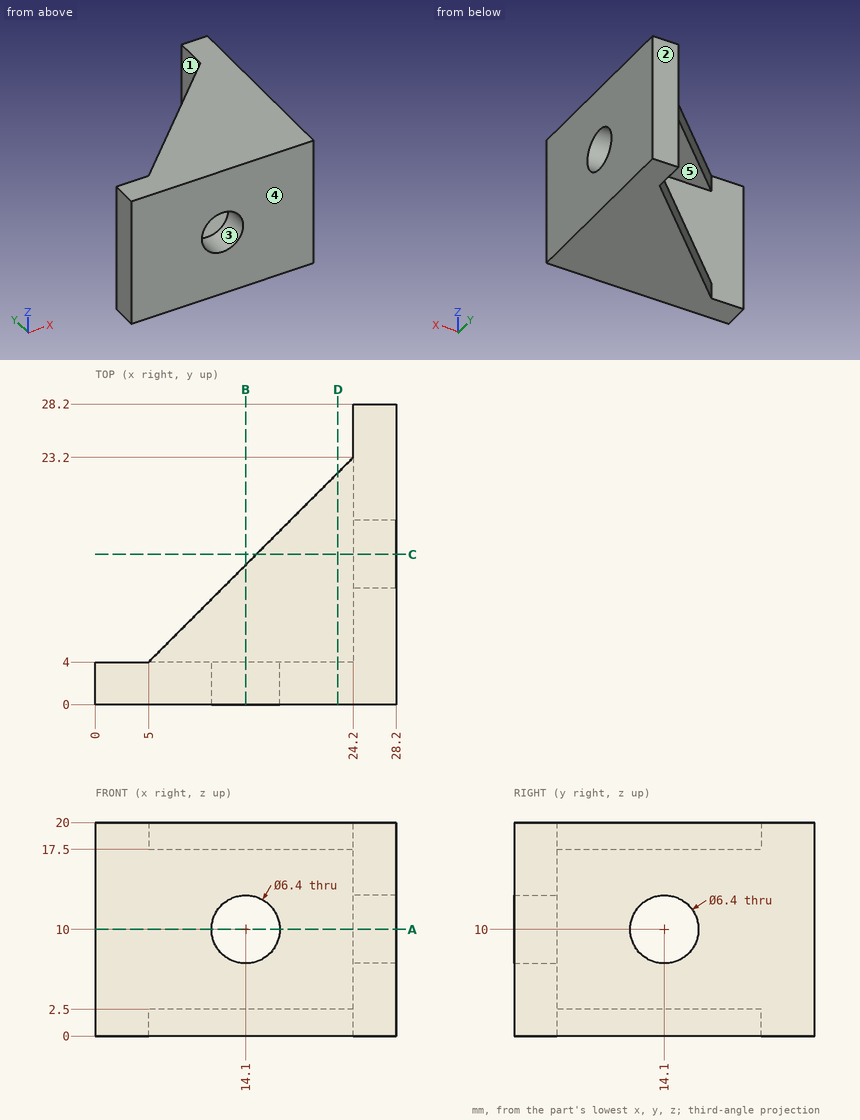
Can you work these out from the drawing? Everything is in mm from the part's minimum corner. A direction names the side the tool comes from. Round coordinates to 2 decimals unless told otherwise and drop trailing zeros. Loops run counter-clockwise (first coordinate to the right, second up) from the corner with the lowest first, then second, coordinate; pieces in that order, holes last. Notation, with made-up numbers: (14, 15) - (53, 15) arc R30 ccw to (53, 42) - close; hole circle Ø6 at (-1, 17.25). An arc over 180 degrees is marked (long way). Answer in a Markdown table with one row per item. Add a question column.
Q1. I want a section at A-A on z = 10. List the corners of the cut face in (x, y) for me, and give its area (3 significant figures).
Q2. We'd pull the mould along X, two halves only. Please class the marked faces 1, 2 and 3: pulls with the +X half, pulls with the -X half, needs draft (parallel to the pull), parting line crosses it, or undercut.
Q3. Which directions (+Z, -Z, +X, -X, +Y, -Y) give clear straight access to the entire face, cutting with the end or side of a thin tool? Please do the marked faces 4 and 5.
Q4. I want a section at D-D on x = 22.75. List the corners of the cut face in (y, z) for me.
Q5. For pin 1 Ø2 at (y, z) = (12, 4.5) entering from -X; pin 2 Ø3 at (x, z) = (10, 3) entering from +Y; pin 3 Ø6 at (x, z) = (9.5, 16) entering from +Y; pin 4 Ø6 at (x, y) = (13, 13) entering from +Z, each with a flat end and sliding along its axis, tell me the tip position at first contact or that it passes through.
Q6. I want a section at B-B on x = 14.1. List the corners of the cut face in (y, z) for me.
Q7. I need wall thicknesses on L1, parallel to Z at x = 25.6, y = 14.1; L2, parallel to Y at x = 25.8, z = 10; L3, parallel to Z at x = 9.5, y = 6.5. Which ranges of each line are inside material? Lowest first, please.
Q8. I want a section at C-C on y = 14.1. List the corners of the cut face in (x, z) for me, and give its area (3 significant figures).
A:
| question | item | result |
|---|---|---|
| 1 | outline | (0, 0) - (10.9, 0) - (10.9, 4) - (0, 4) - close; (17.3, 0) - (28.2, 0) - (28.2, 10.9) - (24.2, 10.9) - (24.2, 4) - (17.3, 4) - close; (24.2, 17.3) - (28.2, 17.3) - (28.2, 28.2) - (24.2, 28.2) - close |
| 1 | area | 158 mm^2 |
| 2 | face 1 | pulls with the -X half |
| 2 | face 2 | needs draft |
| 2 | face 3 | undercut |
| 3 | face 4 | +Z, -Z, +X, -X, -Y |
| 3 | face 5 | -X, +Y |
| 4 | outline | (0, 0) - (21.75, 0) - (21.75, 2.5) - (4, 2.5) - (4, 17.5) - (21.75, 17.5) - (21.75, 20) - (0, 20) - close |
| 5 | pin 1 | x = 24.2 |
| 5 | pin 2 | y = 10.41 |
| 5 | pin 3 | y = 11.1 |
| 5 | pin 4 | z = 20 |
| 6 | outline | (0, 0) - (13.1, 0) - (13.1, 2.5) - (4, 2.5) - (4, 6.8) - (0, 6.8) - close; (0, 13.2) - (4, 13.2) - (4, 17.5) - (13.1, 17.5) - (13.1, 20) - (0, 20) - close |
| 7 | L1 | 0 to 6.8, 13.2 to 20 |
| 7 | L2 | 0 to 10.9, 17.3 to 28.2 |
| 7 | L3 | 0 to 2.5, 17.5 to 20 |
| 8 | outline | (15.1, 0) - (28.2, 0) - (28.2, 6.8) - (24.2, 6.8) - (24.2, 2.5) - (15.1, 2.5) - close; (15.1, 17.5) - (24.2, 17.5) - (24.2, 13.2) - (28.2, 13.2) - (28.2, 20) - (15.1, 20) - close |
| 8 | area | 99.9 mm^2 |
